Here's how the part is built. I have some questions about the finished solid (model axes, mm). Face numbers are marked on the shaded views. Round coordinates to 2 decimals unless told otherwise and drop trailing zeros. Write each loop counter-clockwise with the first axis right and the second up, starting at its lowest first coordinate (ties: lowest second). Pieces come first, ordered by that corner, then holes. Notation, with made-up numbers: (7, 53) -> (58, 53) arc R35 cw to (58, 88) -> close; hole circle Ø3 at (78, -14.5). An arc over 180 degrees is marked (long way). Answer as CSV lines item,"result".
from build123d import *

# Parameters (mm, degrees)
SALIENTE_EXTRUIR1_DEPTH = 2.5
SALIENTE_EXTRUIR2_DEPTH = 45
CROQUIS17_R             = 2
CROQUIS17_R_2           = 1.5
CORTAR_EXTRUIR1_DEPTH   = 45
CROQUIS18_R             = 0.5
SALIENTE_EXTRUIR3_DEPTH = 3
CROQUIS19_W             = 84
CROQUIS19_H             = 2
CORTAR_EXTRUIR2_DEPTH   = 10
CROQUIS24_W             = 0.024080101
CROQUIS24_H             = 2
CORTAR_EXTRUIR11_DEPTH  = 2
CROQUIS30_W             = 1
CROQUIS30_H             = 1
CORTAR_EXTRUIR12_DEPTH  = 101
CROQUIS32_W             = 1
CROQUIS32_H             = 79.482316352
CORTAR_EXTRUIR13_DEPTH  = 1
CROQUIS33_W             = 1
CROQUIS33_H             = 1
CORTAR_EXTRUIR14_DEPTH  = 1
CROQUIS35_R             = 0.5
SALIENTE_EXTRUIR4_DEPTH = 3
CROQUIS37_R             = 0.5
CORTAR_EXTRUIR15_DEPTH  = 4
CROQUIS38_R             = 0.5
CORTAR_EXTRUIR16_DEPTH  = 4
CORTAR_EXTRUIR17_DEPTH  = 1
CROQUIS40_R             = 7.515901536
CROQUIS40_R_2           = 3.728280466
CROQUIS40_R_3           = 3.722695871
CORTAR_EXTRUIR19_DEPTH  = 0.9
CROQUIS41_R             = 0.5
SALIENTE_EXTRUIR5_DEPTH = 3
CROQUIS42_R             = 0.5
SALIENTE_EXTRUIR6_DEPTH = 3
CROQUIS45_R             = 0.5
CORTAR_EXTRUIR22_DEPTH  = 4
CROQUIS46_R             = 0.5
CORTAR_EXTRUIR23_DEPTH  = 4


with BuildPart() as part:
    # Croquis15 → Saliente-Extruir1 (new body)
    with BuildSketch(Plane.XY):
        Polygon((0, 80), (86, 80), (86.987170897, -1.494021214), (0.493585448, -0.747010607), align=None)
    extrude(amount=SALIENTE_EXTRUIR1_DEPTH)

    # Croquis16 → Saliente-Extruir2 (add)
    with BuildSketch(Plane.XY.offset(2.5)):
        Polygon((0, 80), (0.01204005, 78), (84.024080101, 78), (84.986811751, -1.476485582), (86.987170897, -1.494021214), (86, 80), align=None)
    extrude(amount=SALIENTE_EXTRUIR2_DEPTH)

    # Croquis17 → Cortar-Extruir1 (cut)
    with BuildSketch(Plane.XY.offset(2.5)):
        with Locations((79.072166937, 74)):
            Circle(CROQUIS17_R)
        with Locations((72.120400503, 63)):
            Circle(CROQUIS17_R_2)
    extrude(amount=-CORTAR_EXTRUIR1_DEPTH, mode=Mode.SUBTRACT)

    # Croquis18 → Saliente-Extruir3 (add)
    with BuildSketch(Plane(origin=(-0.006414337, -0.742692308, 0), x_dir=(0.9999627066458414, -0.008636279148040384, 0), z_dir=(-0.008636279148040384, -0.9999627066458414, 0))):
        with Locations(Location((2.500018433, 1.25, 0), (0, 0, 180))):
            Circle(CROQUIS18_R)
        with Locations(Location((85.996829638, 1.25, 0), (0, 0, 180))):
            Circle(CROQUIS18_R)
        with Locations(Location((22.500018433, 1.25, 0), (0, 0, 180))):
            Circle(CROQUIS18_R)
        with Locations(Location((65.996829638, 1.25, 0), (0, 0, 180))):
            Circle(CROQUIS18_R)
        with Locations(Location((43.496829638, 1.25, 0), (0, 0, 180))):
            Circle(CROQUIS18_R)
    extrude(amount=SALIENTE_EXTRUIR3_DEPTH)

    # Croquis19 → Cortar-Extruir2 (cut)
    with BuildSketch(Plane(origin=(0, 80, 0), x_dir=(1, 0, 0), z_dir=(0, 1, 0))):
        with Locations((42, -46.5)):
            Rectangle(CROQUIS19_W, CROQUIS19_H)
    extrude(amount=-CORTAR_EXTRUIR2_DEPTH, mode=Mode.SUBTRACT)

    # Croquis24 → Cortar-Extruir11 (cut)
    with BuildSketch(Plane.XY.offset(47.5)):
        with Locations((84.012040051, 79)):
            Rectangle(CROQUIS24_W, CROQUIS24_H)
    extrude(amount=-CORTAR_EXTRUIR11_DEPTH, mode=Mode.SUBTRACT)

    # Croquis30 → Cortar-Extruir12 (cut)
    with BuildSketch(Plane(origin=(0, 80, 0), x_dir=(1, 0, 0), z_dir=(0, 1, 0))):
        with Locations((84.524080101, -46)):
            Rectangle(CROQUIS30_W, CROQUIS30_H)
    extrude(amount=-CORTAR_EXTRUIR12_DEPTH, mode=Mode.SUBTRACT)

    # Croquis32 → Cortar-Extruir13 (cut)
    with BuildSketch(Plane(origin=(84.956460397, 1.029112859, 0), x_dir=(0, 0, 1), z_dir=(-0.9999266406620362, -0.01211252633991657, 0))):
        with Locations((46, 37.235375912)):
            Rectangle(CROQUIS32_W, CROQUIS32_H)
    extrude(amount=-CORTAR_EXTRUIR13_DEPTH, mode=Mode.SUBTRACT)

    # Croquis33 → Cortar-Extruir14 (cut)
    with BuildSketch(Plane(origin=(-0.006411756, -0.731414451, 0), x_dir=(0.9999615787185102, -0.008765904789859459, 0), z_dir=(-0.008765904789859457, -0.9999615787185101, 0))):
        with Locations((85.496489181, 46)):
            Rectangle(CROQUIS33_W, CROQUIS33_H)
    extrude(amount=-CORTAR_EXTRUIR14_DEPTH, mode=Mode.SUBTRACT)

    # Croquis35 → Saliente-Extruir4 (add)
    with BuildSketch(Plane(origin=(-0.006411756, -0.731414451, 0), x_dir=(0.9999615787185102, -0.008765904789859459, 0), z_dir=(-0.008765904789859457, -0.9999615787185101, 0))):
        with Locations(Location((85.996707183, 37.5, 0), (0, 0, 180))):
            Circle(CROQUIS35_R)
    extrude(amount=SALIENTE_EXTRUIR4_DEPTH)

    # Croquis37 → Cortar-Extruir15 (cut)
    with BuildSketch(Plane(origin=(-0.006411756, -0.731414451, 0), x_dir=(0.9999615787185102, -0.008765904789859459, 0), z_dir=(-0.008765904789859457, -0.9999615787185101, 0))):
        with Locations((85.996925186, 9.5)):
            Circle(CROQUIS37_R)
    extrude(amount=-CORTAR_EXTRUIR15_DEPTH, mode=Mode.SUBTRACT)

    # Croquis38 → Cortar-Extruir16 (cut)
    with BuildSketch(Plane(origin=(-0.006414337, -0.742692308, 0), x_dir=(0.9999627066458414, -0.008636279148040382, 0), z_dir=(-0.008636279148040382, -0.9999627066458414, 0))):
        with Locations((12.500018433, 1.25)):
            Circle(CROQUIS38_R)
        with Locations((32.500018433, 1.25)):
            Circle(CROQUIS38_R)
        with Locations((55.000018433, 1.25)):
            Circle(CROQUIS38_R)
        with Locations((77.000018433, 1.25)):
            Circle(CROQUIS38_R)
    extrude(amount=-CORTAR_EXTRUIR16_DEPTH, mode=Mode.SUBTRACT)

    # Croquis39 → Cortar-Extruir17 (cut)
    # profile 1 of 3: a face of its own
    with BuildSketch(Plane(origin=(0, 80, 0), x_dir=(1, 0, 0), z_dir=(0, 1, 0))):
        Polygon((42.740086015, -38), (27.970855246, -6), (31.092650117, -6), (35.823419348, -16.256410256), (50.329829605, -16.256410256), (55.19521422, -6), (58.329829605, -6), (43.150342425, -38), align=None)
        Polygon((42.977265502, -31.762820513), (48.772137297, -19.538461538), (37.336239861, -19.538461538), align=None, mode=Mode.SUBTRACT)
    # profile 2 of 3: a face of its own
    with BuildSketch(Plane(origin=(0, 80, 0), x_dir=(1, 0, 0), z_dir=(0, 1, 0))):
        Polygon((29.447778323, -34.717948718), (29.447778323, -38), (12.627265502, -38), (12.627265502, -34.717948718), (19.601624476, -34.717948718), (19.601624476, -6), (22.473419348, -6), (22.473419348, -34.717948718), align=None)
    # profile 3 of 3: a face of its own
    with BuildSketch(Plane(origin=(0, 80, 0), x_dir=(1, 0, 0), z_dir=(0, 1, 0))):
        Polygon((9.591368066, -38), (6.719573194, -38), (6.719573194, -9.282051282), (-5.588119113, -9.282051282), (-5.588119113, -6), (9.591368066, -6), align=None)
    extrude(amount=-CORTAR_EXTRUIR17_DEPTH, mode=Mode.SUBTRACT)

    # Croquis40 → Cortar-Extruir19 (cut)
    # profile 1 of 3: a face of its own
    with BuildSketch(Plane(origin=(86.956313679, 1.053337912, 0), x_dir=(0, 0, -1), z_dir=(0.9999266406620362, 0.012112526339916658, 0))):
        with Locations(Location((-21.026467212, 22.472656931, 0), (0, 0, 90))):
            Circle(CROQUIS40_R)
        with Locations(Location((-21.026467212, 22.472656931, 0), (0, 0, 90))):
            Circle(CROQUIS40_R_2, mode=Mode.SUBTRACT)
    # profile 2 of 3: a face of its own
    with BuildSketch(Plane(origin=(86.956313679, 1.053337912, 0), x_dir=(0, 0, -1), z_dir=(0.9999266406620362, 0.012112526339916658, 0))):
        with BuildLine():
            Line((-21.026467212, -0.713555766), (-33.411935882, -0.713555766))
            Line((-33.411935882, -0.713555766), (-33.411935882, 3.110384386))
            Line((-33.411935882, 3.110384386), (-27.461333641, 3.110384386))
            ThreePointArc((-27.461333641, 3.110384386), (-17.28380692, 12.910750348), (-21.026467212, -0.713555766))
        make_face()
        with Locations(Location((-21.026467212, 6.612660391, 0), (0, 0, 90))):
            Circle(CROQUIS40_R_3, mode=Mode.SUBTRACT)
    # profile 3 of 3: a face of its own
    with BuildSketch(Plane(origin=(86.956313679, 1.053337912, 0), x_dir=(0, 0, -1), z_dir=(0.9999266406620362, 0.012112526339916658, 0))):
        with BuildLine():
            Line((-24.518011858, 36.31920775), (-24.518011858, 41.791750463))
            Line((-24.518011858, 41.791750463), (-27.82511635, 41.791750463))
            Line((-27.82511635, 41.791750463), (-27.82511635, 36.31920775))
            Line((-27.82511635, 36.31920775), (-33.411935882, 36.31920775))
            Line((-33.411935882, 36.31920775), (-33.411935882, 32.706016439))
            Line((-33.411935882, 32.706016439), (-27.82511635, 32.706016439))
            Line((-27.82511635, 32.706016439), (-27.82511635, 30.846665037))
            Line((-27.82511635, 30.846665037), (-24.518011858, 30.846665037))
            Line((-24.518011858, 30.846665037), (-24.518011858, 32.706016439))
            Line((-24.518011858, 32.706016439), (-19.754047189, 32.706016439))
            ThreePointArc((-19.754047189, 32.706016439), (-15.568413472, 34.624986495), (-13.859170054, 38.900552261))
            Line((-13.859170054, 38.900552261), (-13.859170054, 41.791750463))
            Line((-13.859170054, 41.791750463), (-17.451500124, 41.791750463))
            Line((-17.451500124, 41.791750463), (-17.451500124, 38.573932348))
            ThreePointArc((-17.451500124, 38.573932348), (-18.28309704, 37.120113126), (-19.754047189, 36.31920775))
            Line((-19.754047189, 36.31920775), (-24.518011858, 36.31920775))
        make_face()
    extrude(amount=-CORTAR_EXTRUIR19_DEPTH, mode=Mode.SUBTRACT)

    # Croquis41 → Saliente-Extruir5 (add)
    with BuildSketch(Plane(origin=(0.489000895, 0.002989135, 0), x_dir=(0, 0, 1), z_dir=(-0.9999813177309185, -0.006112625388175003, 0))):
        with Locations(Location((1.25, 78.998505418, 0), (0, 0, 90))):
            Circle(CROQUIS41_R)
        with Locations(Location((1.25, 58.998505418, 0), (0, 0, 90))):
            Circle(CROQUIS41_R)
        with Locations(Location((1.25, 38.998505418, 0), (0, 0, 90))):
            Circle(CROQUIS41_R)
        with Locations(Location((1.25, 18.998505418, 0), (0, 0, 90))):
            Circle(CROQUIS41_R)
    extrude(amount=SALIENTE_EXTRUIR5_DEPTH)

    # Croquis42 → Saliente-Extruir6 (add)
    with BuildSketch(Plane(origin=(0.481584557, 0.002899151, 0), x_dir=(0, 0, 1), z_dir=(-0.9999818801412468, -0.006019916044037572, 0))):
        with Locations(Location((43.5, 78.998532291, 0), (0, 0, 90))):
            Circle(CROQUIS42_R)
        with Locations(Location((23.5, 78.998532291, 0), (0, 0, 90))):
            Circle(CROQUIS42_R)
    extrude(amount=SALIENTE_EXTRUIR6_DEPTH)

    # Croquis45 → Cortar-Extruir22 (cut)
    with BuildSketch(Plane(origin=(0.481584557, 0.002899151, 0), x_dir=(0, 0, 1), z_dir=(-0.9999818801412468, -0.006019916044037572, 0))):
        with Locations(Location((33.5, 78.998532291, 0), (0, 0, 270))):
            Circle(CROQUIS45_R)
        with Locations(Location((13.5, 78.998532291, 0), (0, 0, 270))):
            Circle(CROQUIS45_R)
    extrude(amount=-CORTAR_EXTRUIR22_DEPTH, mode=Mode.SUBTRACT)

    # Croquis46 → Cortar-Extruir23 (cut)
    with BuildSketch(Plane(origin=(0.489000895, 0.002989135, 0), x_dir=(0, 0, 1), z_dir=(-0.9999813177309185, -0.006112625388175003, 0))):
        with Locations(Location((1.25, 68.998505418, 0), (0, 0, 270))):
            Circle(CROQUIS46_R)
        with Locations(Location((1.25, 48.998505418, 0), (0, 0, 270))):
            Circle(CROQUIS46_R)
        with Locations(Location((1.25, 28.998505418, 0), (0, 0, 270))):
            Circle(CROQUIS46_R)
        with Locations(Location((1.25, 8.998505418, 0), (0, 0, 270))):
            Circle(CROQUIS46_R)
    extrude(amount=-CORTAR_EXTRUIR23_DEPTH, mode=Mode.SUBTRACT)


solid = part.part
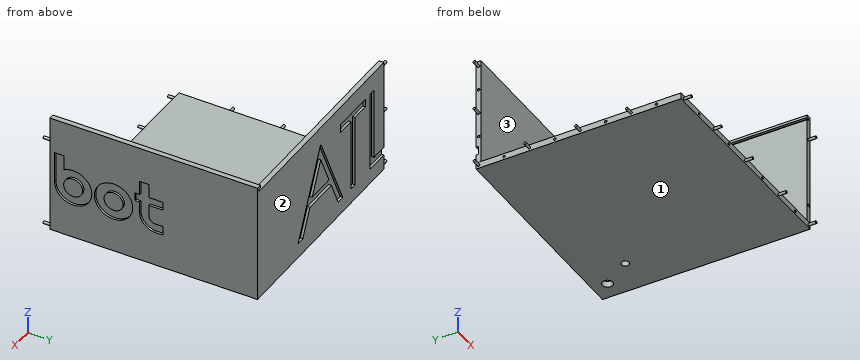
Item 1: If we mould it in two halves opening along Y, with no side actions, what happens to the marked faces 1, 2 and 3? For each: pulls with the +Y half, pulls with the -Y half, needs draft (parallel to the pull), parting line crosses it, or undercut.
Results found:
face 1,"needs draft"
face 2,"pulls with the +Y half"
face 3,"pulls with the -Y half"
Item 2: Will these pins go through, and if not, where does the flat tip stop? pin 1 (1 mm diameter, centred on x = 50, y = 42, fed in from +Z); pin 2 (12 mm diameter, centred on y = 17, z = 37, fed in from +X); pin 3 (0.5 mm diameter, centred on x = 44.5, y = 79.5, fed in from +Z).
Results found:
pin 1,"stops at z = 2.5"
pin 2,"stops at x = 86.84"
pin 3,"stops at z = 45.5"
Item 3: Suppose I cut it at C-C, the plane y = 74. List the corners of the cut face in (x, z) for me, then the cut area to 3 significant figures.
Results found:
outline,"(0.04, 0) -> (77.07, 0) -> (77.07, 2.5) -> (0.04, 2.5) -> close; (81.07, 0) -> (86.07, 0) -> (86.07, 47.5) -> (84.07, 47.5) -> (84.07, 46.5) -> (85.07, 46.5) -> (85.07, 45.5) -> (84.07, 45.5) -> (84.07, 2.5) -> (81.07, 2.5) -> close"
area,"294 mm²"
Item 4: Suppose I cut it at B-B, the plane z = 41. List the corners of the cut face in (x, y) for me, then the cut area to 3 significant figures.
Results found:
outline,"(0, 80) -> (0.01, 78) -> (84.02, 78) -> (84.99, -1.48) -> (86.99, -1.49) -> (86, 80) -> close"
area,"331 mm²"
Item 5: Suppose I cut it at D-D, the plane x = 39. List the corners of the cut face in (y, z) for me, then the cut area to 3 significant figures.
Results found:
outline,"(-1.08, 0) -> (80, 0) -> (80, 16.26) -> (79, 16.26) -> (79, 19.54) -> (80, 19.54) -> (80, 23.14) -> (79, 23.14) -> (79, 29.9) -> (80, 29.9) -> (80, 45.5) -> (78, 45.5) -> (78, 2.5) -> (-1.08, 2.5) -> close"
area,"279 mm²"
Item 6: I need wall thicknesses on L1, parallel to Y at x = 23.5, z = 38.5; L2, parallel to Z at x = 40, y = 74; L3, parallel to X at y = 0.5, z = 3.5. Which ranges of each line are inside material? Lowest first, please.
Results found:
L1,"y = 78 to 80"
L2,"z = 0 to 2.5"
L3,"x = 84.96 to 86.96"
Item 7: Suppose I cut it at A-A, the plane x = 72. List the corners of the cut face in (y, z) for me.
Results found:
outline,"(-1.36, 0) -> (61.5, 0) -> (61.5, 2.5) -> (-1.36, 2.5) -> close; (64.5, 0) -> (80, 0) -> (80, 45.5) -> (78, 45.5) -> (78, 2.5) -> (64.5, 2.5) -> close"
